Could you check a few things on this model? Use its own coordinates, in mm. Face numbers are marked on the shaded views. A direction names the side the tool comes from. Give positions to 0.01 mm unless a question says otherwise; leave off trailing zeros. Write each loop counter-clockwise with the first axis right and the second up, starting at its lowest first coordinate (ties: lowest second). Pieces come first, ordered by that corner, then holes. Notation, with made-up numbers: M -19.75,46.5 L -15.75,46.5 A32 ccw -15.75,85.5 Z; hole C -13.5,25.25 d6. An arc over 180 degrees is marked long. Use one line per item in the form item = value.
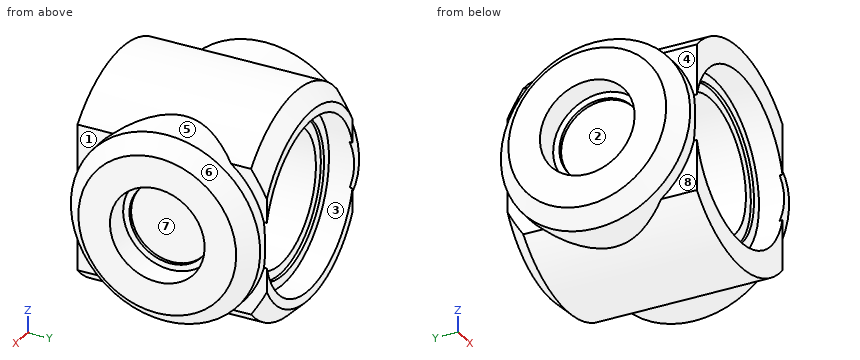
from build123d import *

# Parameters (mm, degrees)
BOSS_EXTRUDE1_DEPTH  = 15
F_2_5MM_CHAMFER_SIZE = 2.5


with BuildPart() as part:
    # Sketch3 → Revolve1 (revolve)
    with BuildSketch(Plane(origin=(0, 0, 0), x_dir=(1, 0, 0), z_dir=(0, 1, 0))):
        Polygon((0, 0), (-13, 0), (-13, 6.5), (-13.5, 6.5), (-13.5, 7.5), (-17.5, 7.5), (-17.5, 15), (0, 15), align=None)
    revolve1 = revolve(axis=Axis((0, 0, 0), (-1, 0, 0)))

    # Mirror1: Revolve1 across plane
    add(revolve1.mirror(Plane(origin=(0, 0, 0), x_dir=(0, 0, 1), z_dir=(1, 0, 0))))

    # Sketch6 → Boss-Extrude1 (add, symmetric)
    with BuildSketch(Plane(origin=(0, 0, 0), x_dir=(1, 0, 0), z_dir=(0, 1, 0))):
        with BuildLine():
            ThreePointArc((12.993588105, 11.722485579), (0, 17.5), (-12.993588105, 11.722485579))
            Line((-12.993588105, 11.722485579), (-12.993588105, -11.722485579))
            ThreePointArc((-12.993588105, -11.722485579), (0, -17.5), (12.993588105, -11.722485579))
            Line((12.993588105, -11.722485579), (12.993588105, 11.722485579))
        make_face()
    extrude(amount=BOSS_EXTRUDE1_DEPTH, both=True)

    # Sketch8 → Cut-Revolve1 (revolve, cut)
    with BuildSketch(Plane.XY, mode=Mode.PRIVATE) as cut_revolve1_sk:
        Polygon((0, -15), (13.5, -15), (13.5, -11), (12, -11), (12, -10.5), (10.5, -10.5), (10.5, 10.5), (12, 10.5), (12, 11), (13.5, 11), (13.5, 15), (0, 15), align=None)
    revolve(cut_revolve1_sk.sketch.rotate(Axis((0, 15, 0), (0, -1, 0)), 90), axis=Axis((0, 15, 0), (0, -1, 0)), mode=Mode.SUBTRACT)

    # 2,5mm Chamfer
    f_2_5mm_chamfer_edges = [part.edges().sort_by_distance(p)[0] for p in [
        (-17.5, 0, 15),
        (17.5, 0, 15),
        (0, 15, 17.5),
        (0, 15, -17.5),
    ]]
    chamfer(f_2_5mm_chamfer_edges, length=F_2_5MM_CHAMFER_SIZE)


solid = part.part
1) Thinking about a two-plate mould opening in Z: for the marked faces 6, 7 and 8, which applies, released by +Z, released by -Z, zero draft, split by the parting line, or undercut?
Checked values:
face_6 = split by the parting line
face_7 = undercut
face_8 = zero draft
2) For the marked faces 1, 2, 3, 4 and 5, which set-ups out of +Z, -Z, +X, -X, +Y, -Y let a thin tool reach every point of the face, with its end or its side?
Checked values:
face_1 = +Z, +X, -Y
face_2 = -X
face_3 = +Y
face_4 = +Z, -X, -Y
face_5 = +X
3) For pin 1 Ø6 at (x, y) = (13.5, -6.5) entering from -Z; pin 2 Ø1.7 at (y, z) = (11, -9) entering from +X; pin 3 Ø12 at (y, z) = (0, 0) entering from -X; pin 4 Ø12 at (x, z) = (3, 1) entering from -Y, each with a flat end and sliding along its axis, tell me the tip position at first contact or that it passes through.
Checked values:
pin_1 = -14.59
pin_2 = 16.64
pin_3 = -13
pin_4 = through
4) If I drill on L1, parallel to X at y = -10, z = 0; L2, parallel to Z at x = -14.8, y = 0; L3, parallel to Y at x = -14.5, z = -0.5, over which ranges is the centre line in solid material (lowest first)?
Checked values:
L1 = -17.5 to -10.5, 10.5 to 17.5
L2 = -15 to -7.5, 7.5 to 15
L3 = -14.99 to -7.48, 7.48 to 14.99
5) I want a section at B-B, the plane x = 0. Please give me the cut outline in (y, z), plus the area to 3 significant figures.
Checked values:
outline = M -15,-17.5 L 12.5,-17.5 L 15,-15 L 15,-13.5 L 11,-13.5 L 11,-12 L 10.5,-12 L 10.5,-10.5 L -10.5,-10.5 L -10.5,-12 L -11,-12 L -11,-13.5 L -15,-13.5 Z; M -15,13.5 L -11,13.5 L -11,12 L -10.5,12 L -10.5,10.5 L 10.5,10.5 L 10.5,12 L 11,12 L 11,13.5 L 15,13.5 L 15,15 L 12.5,17.5 L -15,17.5 Z
area = 363 mm2
